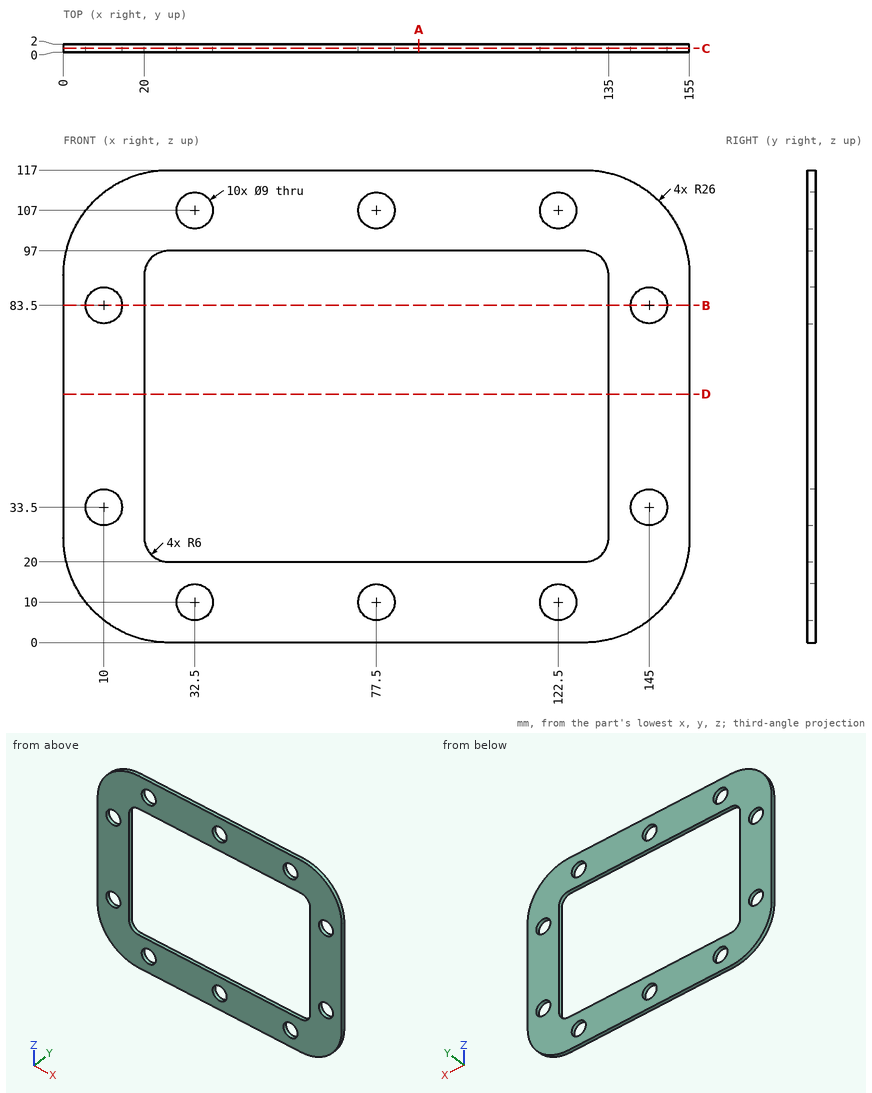
For this review, use the dimensioned drawing (mm, ordinates from the lowest corner) and the shaded views. Give positions to 0.01 mm unless a question says otherwise; leave off trailing zeros. Write each loop counter-clockwise with the first axis right and the second up, starting at its lowest first coordinate (ties: lowest second). Pieces come first, ordered by that corner, then holes. Notation, with made-up numbers: M 66,-36.5 L 80,-36.5 A21 cw 80,-17.5 Z; hole C 22,10.5 d5. An arc over 180 degrees is marked long. Answer as a JSON object with one key per item and string values. Group by question number.
1) For line 1 along X through (y, z) = (1.1, 10); line 2 along Z through (x, y) = (122, 0.65); line 3 along Z through (x, y) = (40.5, 1.1), list the stretches that pass through material, from the lowest coordinate up.
2) We need section D-D (z = 61.5). Give the boundary of the cut face in (x, y), and give its area (3 significant figures).
3) Clearance check with a flat-ended pin moving along its axis: pin 1 Ø8 at (x, z) = (10, 83.5) entering from +Y. State where the tip first meets the part, or that it passes through.
4) We need section A-A (x = 88). Give the boundary of the cut face in (y, z), and give its area (3 significant figures).
5) We need section B-B (z = 83.5). Give the boundary of the cut face in (x, y), and give its area (3 significant figures).
6) We need section C-C (y = 0.9). Count the separate pieces of the cut face and the enclosed holes in it, and give its area (3 significant figures).
Answer key:
{
 "1": {"line 1": "x = 5.51 to 28, 37 to 73, 82 to 118, 127 to 149.49", "line 2": "z = 0 to 5.53, 14.47 to 20, 97 to 102.53, 111.47 to 117", "line 3": "z = 0 to 20, 97 to 117"},
 "2": {"outline": "M 0,0 L 20,0 L 20,2 L 0,2 Z; M 135,0 L 155,0 L 155,2 L 135,2 Z", "area": "80.0 mm²"},
 "3": {"pin 1": "passes through"},
 "4": {"outline": "M 0,0 L 2,0 L 2,20 L 0,20 Z; M 0,97 L 2,97 L 2,117 L 0,117 Z", "area": "80.0 mm²"},
 "5": {"outline": "M 0,0 L 5.5,0 L 5.5,2 L 0,2 Z; M 14.5,0 L 20,0 L 20,2 L 14.5,2 Z; M 135,0 L 140.5,0 L 140.5,2 L 135,2 Z; M 149.5,0 L 155,0 L 155,2 L 149.5,2 Z", "area": "44.0 mm²"},
 "6": {"separate pieces": "1", "enclosed holes": "11", "area": "8,090 mm²"}
}
